Here's how the part is built. I have some questions about the finished solid (model axes, mm). A direction names the side the tool comes from. Coordinates: 2 decimals unless noted, no trailing zeros. Write each loop counter-clockwise with the first axis right and the second up, starting at its lowest first coordinate (ties: lowest second). Pieces come first, ordered by that corner, then holes.
Item 1: If we mould it in two halves opening along X, with no side actions, what happens to faces 3 (the face through (-44, 79.79, -107.51)), 4 (the face through (0, 110.5, -108)), 5 (the face through (90.29, -1.3, -107.51))? For each: pulls with the +X half, pulls with the -X half, needs draft (parallel to the pull), parting line crosses it, or undercut.
Item 2: I want a section at D-D (z = -106.45). Count the separate pieces of the cut face and the enclosed holes in it, and give its area (3 significant figures).
Item 3: I want a section at C-C (x = 53.5). Please give me the cut outline in (y, z) (3 decimals), and give its area (3 significant figures).
Item 4: I want a section at B-B (y = -100). Please give me the cut outline in (x, z) (3 decimals).
Item 5: Please list where these lines run through material, in increasing order: line 1 (Y direction, x = -20, z = -108.55); line 2 (Y direction, x = -30, z = -108.4); line 3 (Y direction, x = 0, z = -108.3).
Item 6: I'm going to push flat-ended pins straight in: P1, Ø4.5, axis at x = -20, y = -100, coming from the -Z side; P2, Ø1.4, axis at y = 103.5, z = -107.5, coming from the +X side; P3, Ø1.5, axis at y = -88, z = -107, coming from the +X side. Where does each tip first touch, or does it pass through?
Item 7: I want a section at A-A (x = 0). Please give me the cut outline in (y, z) (3 decimals).
Item 8: For faces 1 (the face through (-34, 77, -105.105)), 2 (the face through (0, 89.5, -108)), which set-ups out of +Z, -Z, +X, -X, +Y, -Y let a thin tool reach every point of the face, with its end or its side?
from build123d import *

# Parameters (mm, degrees)
SKETCH2_R           = 3.75
SKETCH2_R_2         = 82.8
BOSS_EXTRUDE1_DEPTH = 4.7498


with BuildPart() as part:
    # Sketch2 → Boss-Extrude1 (new body)
    with BuildSketch(Plane.XY.offset(-109.855)):
        with BuildLine():
            Line((34.829629131, -111.294095226), (42.367226853, -83.16339756))
            ThreePointArc((42.367226853, -83.16339756), (44.027245948, -79.750573703), (46.839397866, -77.202077741))
            ThreePointArc((46.839397866, -77.202077741), (90.3, 0), (46.839397866, 77.202077741))
            ThreePointArc((46.839397866, 77.202077741), (44.027245948, 79.750573703), (42.367226853, 83.16339756))
            Line((42.367226853, 83.16339756), (34.829629131, 111.294095226))
            ThreePointArc((34.829629131, 111.294095226), (33.043807145, 113.966766701), (30, 115))
            Line((30, 115), (-30, 115))
            ThreePointArc((-30, 115), (-33.043807145, 113.966766701), (-34.829629131, 111.294095226))
            Line((-34.829629131, 111.294095226), (-42.367226853, 83.16339756))
            ThreePointArc((-42.367226853, 83.16339756), (-44.027245948, 79.750573703), (-46.839397866, 77.202077741))
            ThreePointArc((-46.839397866, 77.202077741), (-90.3, 0), (-46.839397866, -77.202077741))
            ThreePointArc((-46.839397866, -77.202077741), (-44.027245948, -79.750573703), (-42.367226853, -83.16339756))
            Line((-42.367226853, -83.16339756), (-34.829629131, -111.294095226))
            ThreePointArc((-34.829629131, -111.294095226), (-33.043807145, -113.966766701), (-30, -115))
            Line((-30, -115), (30, -115))
            ThreePointArc((30, -115), (33.043807145, -113.966766701), (34.829629131, -111.294095226))
        make_face()
        with Locations((20, -100)):
            Circle(SKETCH2_R, mode=Mode.SUBTRACT)
        with Locations((-20, -100)):
            Circle(SKETCH2_R, mode=Mode.SUBTRACT)
        with Locations((-20, 100)):
            Circle(SKETCH2_R, mode=Mode.SUBTRACT)
        with Locations((20, 100)):
            Circle(SKETCH2_R, mode=Mode.SUBTRACT)
        Circle(SKETCH2_R_2, mode=Mode.SUBTRACT)
        with BuildLine():
            Line((9.5, 89.5), (-9.5, 89.5))
            ThreePointArc((-9.5, 89.5), (-10.207106781, 89.792893219), (-10.5, 90.5))
            Line((-10.5, 90.5), (-10.5, 109.5))
            ThreePointArc((-10.5, 109.5), (-10.207106781, 110.207106781), (-9.5, 110.5))
            Line((-9.5, 110.5), (9.5, 110.5))
            ThreePointArc((9.5, 110.5), (10.207106781, 110.207106781), (10.5, 109.5))
            Line((10.5, 109.5), (10.5, 90.5))
            ThreePointArc((10.5, 90.5), (10.207106781, 89.792893219), (9.5, 89.5))
        make_face(mode=Mode.SUBTRACT)
        with BuildLine():
            Line((9.5, -110.5), (-9.5, -110.5))
            ThreePointArc((-9.5, -110.5), (-10.207106781, -110.207106781), (-10.5, -109.5))
            Line((-10.5, -109.5), (-10.5, -90.5))
            ThreePointArc((-10.5, -90.5), (-10.207106781, -89.792893219), (-9.5, -89.5))
            Line((-9.5, -89.5), (9.5, -89.5))
            ThreePointArc((9.5, -89.5), (10.207106781, -89.792893219), (10.5, -90.5))
            Line((10.5, -90.5), (10.5, -109.5))
            ThreePointArc((10.5, -109.5), (10.207106781, -110.207106781), (9.5, -110.5))
        make_face(mode=Mode.SUBTRACT)
    extrude(amount=BOSS_EXTRUDE1_DEPTH)


solid = part.part
Answer:
1. face 3: pulls with the -X half
1. face 4: undercut
1. face 5: pulls with the +X half
2. separate pieces: 1
2. enclosed holes: 7
2. area: 7,250 mm2
3. outline: (-72.745, -109.855) - (-63.195, -109.855) - (-63.195, -105.105) - (-72.745, -105.105) - close; (63.195, -109.855) - (72.745, -109.855) - (72.745, -105.105) - (63.195, -105.105) - close
3. area: 90.7 mm2
4. outline: (-37.856, -109.855) - (-23.75, -109.855) - (-23.75, -105.105) - (-37.856, -105.105) - close; (-16.25, -109.855) - (-10.5, -109.855) - (-10.5, -105.105) - (-16.25, -105.105) - close; (10.5, -109.855) - (16.25, -109.855) - (16.25, -105.105) - (10.5, -105.105) - close; (23.75, -109.855) - (37.856, -109.855) - (37.856, -105.105) - (23.75, -105.105) - close
5. line 1: y = -115 to -103.75, -96.25 to -80.35, 80.35 to 96.25, 103.75 to 115
5. line 2: y = -115 to -77.17, 77.17 to 115
5. line 3: y = -115 to -110.5, -89.5 to -82.8, 82.8 to 89.5, 110.5 to 115
6. P1: passes through
6. P2: stops at x = 37.11
6. P3: stops at x = 41.27
7. outline: (-115, -109.855) - (-110.5, -109.855) - (-110.5, -105.105) - (-115, -105.105) - close; (-89.5, -109.855) - (-82.8, -109.855) - (-82.8, -105.105) - (-89.5, -105.105) - close; (82.8, -109.855) - (89.5, -109.855) - (89.5, -105.105) - (82.8, -105.105) - close; (110.5, -109.855) - (115, -109.855) - (115, -105.105) - (110.5, -105.105) - close
8. face 1: +Z, +X, -X, +Y, -Y
8. face 2: +Z, -Z
